Solid Edge part; units mm, degrees
sketch "Sketch1" plane through (0, 0, 0) normal (0, -1, 0) x (1, 0, 0)
  line L0 (-100, 125) -> (100, 125)
  line L1 (100, 125) -> (100, -125)
  line L2 (100, -125) -> (-100, -125)
  line L3 (-100, -125) -> (-100, 125)
  dimension "D1" = 100
  dimension "D2" = 100
extrude "Protrusion1" add sketch "Sketch1" along normal mid plane 6
sketch "Sketch2" plane through (0, -3, 0) normal (0, -1, 0) x (1, 0, 0)
  line L0 (-30, 55) -> (30, 55)
  line L1 (30, 55) -> (30, -5)
  line L2 (30, -5) -> (-30, -5)
  line L3 (-30, -5) -> (-30, 55)
  dimension "D1" = 30
  dimension "D2" = 30
extrude "Ausprägung_2" add sketch "Sketch2" along normal blind 35
hole "Bohrung_4" at (20, -38, 45) direction (0, 1, 0) diameter 8 end up to next
hole "Hole1" at (0, -38, 5) direction (0, 1, 0) diameter 8 end up to next
hole "Hole2" at (-20, -38, 45) direction (0, 1, 0) diameter 8 end up to next
sketch "Sketch3" plane through (0, -3, 0) normal (0, -1, 0) x (1, 0, 0)
  circle A0 centre (0, -25) radius 5
extrude "Ausschnitt_1" cut sketch "Sketch3" against normal blind 469.9
sketch "Sketch4" plane through (0, -3, 0) normal (0, -1, 0) x (1, 0, 0)
  line L0 (-4.0233, -22.0313) -> (4.0233, -22.0313)
  line L1 (-80, -125) -> (-4.0233, -22.0313)
  line L2 (-80, -125) -> (80, -125)
  line L3 (80, -125) -> (4.0233, -22.0313)
  dimension "D1" = 80
extrude "Ausschnitt_3" cut sketch "Sketch4" against normal blind 320.675
sketch "Sketch5" plane through (0, -3, 0) normal (0, -1, 0) x (1, 0, 0)
  circle A0 centre (0, 75) radius 5
extrude "Ausschnitt_4" cut sketch "Sketch5" against normal blind 250.825
sketch "Sketch6" plane through (0, -3, 0) normal (0, -1, 0) x (1, 0, 0)
  line L0 (-40, 125) -> (-4.1363, 72.1909)
  line L1 (-4.1363, 72.1909) -> (4.1363, 72.1909)
  line L2 (4.1363, 72.1909) -> (40, 125)
  line L3 (40, 125) -> (-40, 125)
  dimension "D1" = 40
extrude "Ausschnitt_5" cut sketch "Sketch6" against normal blind 673.1
sketch "Sketch7" plane through (0, -3, 0) normal (0, -1, 0) x (0.5937309, 0, 0.8046637)
  line L0 (-127.5561, 30.1567) -> (-26.5002, 30.1567)
  line L1 (-26.5002, 30.1567) -> (19.5431, 64.1303)
  line L2 (19.5431, 64.1303) -> (48.1256, 145.3101)
  line L3 (48.1256, 145.3101) -> (48.1256, 179.0397)
  line L4 (48.1256, 179.0397) -> (-141.6388, 49.5277)
  line L5 (-141.6388, 49.5277) -> (-127.5561, 30.1567)
  dimension "D1" = 127.5561
extrude "Ausschnitt_6" cut sketch "Sketch7" against normal blind 1343.025
sketch "Sketch8" plane through (0, -3, 0) normal (0, -1, 0) x (0.5937309, 0, 0.8046637)
  line L0 (-8.8099, -130.776) -> (20.9983, -34.2164)
  line L1 (20.9983, -34.2164) -> (67.0416, -0.2428)
  line L2 (67.0416, -0.2428) -> (153.0403, 3.1226)
  line L3 (153.0403, 3.1226) -> (159.956, -6.25)
  line L4 (159.956, -6.25) -> (-8.8099, -130.776)
extrude "Ausschnitt_8" cut sketch "Sketch8" against normal blind 660.4
sketch "Sketch9" plane through (100, 0, -104.8674) normal (1, 0, 0) x (0, 0, -1)
  line L0 (-20.1326, 3) -> (20.1326, 3)
  line L1 (20.1326, 3) -> (20.1326, -3)
  line L2 (20.1326, -3) -> (-20.1326, -3)
  line L3 (-20.1326, -3) -> (-20.1326, 3)
  dimension "D1" = 20.1326
  dimension "D2" = 20.1326
extrude "Ausprägung_4" add sketch "Sketch9" along normal blind 35
sketch "Sketch10" plane through (17.5, -3, 0) normal (0, -1, 0) x (-0.5937309, 0, -0.8046637)
  line L0 (19.2002, 116.6944) -> (33.9603, 164.5078)
  line L1 (33.9603, 164.5078) -> (30.8196, 168.7643)
  line L2 (30.8196, 168.7643) -> (-1.5804, 144.8576)
  line L3 (-1.5804, 144.8576) -> (19.2002, 116.6944)
extrude "Ausschnitt_9" cut sketch "Sketch10" against normal blind 101.6
sketch "Sketch11" plane through (-100, 0, -104.8674) normal (-1, 0, 0) x (0, 0, -1)
  line L0 (-20.1326, 3) -> (20.1326, 3)
  line L1 (20.1326, 3) -> (20.1326, -3)
  line L2 (20.1326, -3) -> (-20.1326, -3)
  line L3 (-20.1326, -3) -> (-20.1326, 3)
extrude "Ausprägung_5" add sketch "Sketch11" along normal blind 35
sketch "Sketch12" plane through (-2.6449, -3, 0) normal (0, -1, 0) x (-0.5937309, 0, -0.8046637)
  line L0 (125.9857, -28.0285) -> (176.0256, -28.0285)
  line L1 (176.0256, -28.0285) -> (179.1663, -32.285)
  line L2 (179.1663, -32.285) -> (146.7663, -56.1917)
  line L3 (146.7663, -56.1917) -> (125.9857, -28.0285)
extrude "Ausschnitt_10" cut sketch "Sketch12" against normal blind 34.925
fillet "Verrundung_4" radius 5 4 edges at (40, 0, -3.4188) (40, 0, 53.8018) (-40, 0, -3.4188) (-40, 0, 53.8018)
properties material "Aluminium, 1060"
Here's how the part is built. I have some questions about the finished solid (model axes, mm). A direction names the side the tool comes from. Coordinates: 2 decimals unless noted, no trailing zeros. Order: outer loops, then holes, each group sorted by start corner. A loop starts at its lowest first (then second) coordinate and runs counter-clockwise, first axis right, second up.
Item 1: I need wall thicknesses on probe 1 along Z at (x, y) = (0, -12); probe 2 along Z at (x, y) = (20, -12); probe 3 along Y at (x, z) = (-30.5, 20). Which ranges of each line are inside material? Lowest first, please.
Response values:
probe 1: z = -5 to 1, 9 to 55
probe 2: z = -5 to 41, 49 to 55
probe 3: y = -3 to 3
Item 2: Which directions (+Z, -Z, +X, -X, +Y, -Y) give clear straight access to the entire face, cutting with the end or side of a thin tool? Please do faces 1 (the face through (40, 0, 25)), 2 (the face through (-64.275, -0.042, 89.547)), 3 (the face through (0, -20, -5)), 4 (the face through (21.8, 0, 98.2)).
Response values:
face 1: +X, +Y, -Y
face 2: -X, +Y, -Y
face 3: -Z, +X, -X, -Y
face 4: +Z, +Y, -Y
Item 3: If we section it at C-C, the plane z = 45: List the corners of the cut face in (x, y) for me, then the cut area to 3 significant figures.
Response values:
outline: (-40, -3) - (-30, -3) - (-30, -38) - (-24, -38) - (-24, 3) - (-40, 3) - close; (-16, -38) - (16, -38) - (16, 3) - (-16, 3) - close; (24, -38) - (30, -38) - (30, -3) - (40, -3) - (40, 3) - (24, 3) - close
area: 1,920 mm2
Item 4: Thinking about a two-plate mould opening in X: for faces 5 (the face through (-42.543, -0.042, -74.236)), 6 (the face through (-40, 0, 25)), 7 (the face through (42.543, -0.042, -74.236)), 8 (the face through (0, -38, 25)), which applies, pulls with the +X half, pulls with the -X half, needs draft (parallel to the pull), parting line crosses it, or undercut?
Response values:
face 5: undercut
face 6: pulls with the -X half
face 7: undercut
face 8: needs draft
Item 5: If we section it at D-D, the plane y = -16.5: List the corners of the cut face in (x, z) for me, then the cut area to 3 significant figures.
Response values:
outline: (-30, -5) - (30, -5) - (30, 55) - (-30, 55) - close; hole circle Ø8 at (-20, 45); hole circle Ø8 at (0, 5); hole circle Ø8 at (20, 45)
area: 3,450 mm2
Item 6: If we section it at A-A, the plane x = 0: List the corners of the cut face in (y, z) for me, then the cut area to 3 significant figures.
Response values:
outline: (-38, -5) - (-3, -5) - (-3, -20) - (3, -20) - (3, 1) - (-38, 1) - close; (-38, 9) - (3, 9) - (3, 70) - (-3, 70) - (-3, 55) - (-38, 55) - close
area: 2,310 mm2
Item 7: If we section it at B-B, the plane z = 5: List the corners of the cut face in (x, y) for me.
Response values:
outline: (-40, -3) - (-30, -3) - (-30, -38) - (-4, -38) - (-4, 3) - (-40, 3) - close; (4, -38) - (30, -38) - (30, -3) - (40, -3) - (40, 3) - (4, 3) - close
Item 8: I'm going to push flat-ended pins straight in: pin 1 Ø8 at (y, z) = (-1.5, 23) entering from +X; pin 2 Ø1.5 at (x, y) = (-21, -21) entering from +Z; pin 3 Ø1.5 at (x, z) = (59, -39) entering from -Y; pin 4 Ø13 at (x, z) = (0, 5) entering from +Y. Where does each tip first touch, or does it pass through?
Response values:
pin 1: stops at x = 40
pin 2: stops at z = 55
pin 3: stops at y = -3
pin 4: stops at y = 3
